Here's how the part is built. I have some questions about the finished solid (model axes, mm). A direction names the side the tool comes from. Round coordinates to 2 decimals unless told otherwise and drop trailing zeros. Order: outer loops, then holes, each group sorted by start corner. A loop starts at its lowest first (then second) coordinate and runs counter-clockwise, first axis right, second up. Notation, with made-up numbers: (74, -18) -> (78, -18) arc R26 ccw to (78, 6) -> close; hole circle Ø9 at (53, 59.5). An arc over 180 degrees is marked (long way). One line per item, written item: value.
```python
from build123d import *

# Parameters (mm, degrees)
SKETCH1_W           = 82.0674
SKETCH1_H           = 79.121
SKETCH1_R           = 12.7
SKETCH1_W_2         = 28.575
SKETCH1_H_2         = 58.801
BOSS_EXTRUDE1_DEPTH = 25.4


with BuildPart() as part:
    # Sketch1 → Boss-Extrude1 (new body)
    with BuildSketch(Plane(origin=(0, 0, 0), x_dir=(1, 0, 0), z_dir=(0, 1, 0))):
        with Locations((-41.0337, 39.5605)):
            Rectangle(SKETCH1_W, SKETCH1_H)
        with Locations(Location((-23.495, 54.61, 0), (0, 0, 270))):
            Circle(SKETCH1_R, mode=Mode.SUBTRACT)
        with Locations((-61.4299, 39.5605)):
            Rectangle(SKETCH1_W_2, SKETCH1_H_2, mode=Mode.SUBTRACT)
    extrude(amount=BOSS_EXTRUDE1_DEPTH)


solid = part.part
```
Q1. I want a section at A-A on x = -62. Write out the boundary of the cut face in (y, z).
Answers:
outline: (0, -79.12) -> (25.4, -79.12) -> (25.4, -68.96) -> (0, -68.96) -> close; (0, -10.16) -> (25.4, -10.16) -> (25.4, 0) -> (0, 0) -> close
Q2. Which directions (+Z, -Z, +X, -X, +Y, -Y) give clear straight access to the entire face, cutting with the end or side of a thin tool? Please do faces 5 (the face through (-42, 13, 0)), 6 (the face through (-62, 13, -10.16)).
Answers:
face 5: +Z, +X, -X, +Y, -Y
face 6: +Y, -Y
Q3. I want a section at D-D on y = 16. Write out the boundary of the cut face in (x, z) (3 decimals), then the cut area to 3 significant figures.
Answers:
outline: (-82.067, -79.121) -> (0, -79.121) -> (0, 0) -> (-82.067, 0) -> close; hole (-75.717, -68.961) -> (-47.142, -68.961) -> (-47.142, -10.16) -> (-75.717, -10.16) -> close; hole circle Ø25.4 at (-23.495, -54.61)
area: 4,310 mm2
Q4. For P1, Ø12, axis at x = -38.5, z = -39.5, coming from the -Y side; P2, Ø20.5, axis at x = -23.495, z = -54.61, coming from the +Y side, each with a flat end and sliding along its axis, tell me the tip position at first contact or that it passes through.
Answers:
P1: y = 0
P2: through
Q5. I want a section at C-C on z = -54.61. Write out the boundary of the cut face in (x, y) (3 decimals), then the cut area to 3 significant figures.
Answers:
outline: (-82.067, 0) -> (-75.717, 0) -> (-75.717, 25.4) -> (-82.067, 25.4) -> close; (-47.142, 0) -> (-36.195, 0) -> (-36.195, 25.4) -> (-47.142, 25.4) -> close; (-10.795, 0) -> (0, 0) -> (0, 25.4) -> (-10.795, 25.4) -> close
area: 714 mm2
Q6. I need wall thicknesses on line 1 along X through (y, z) = (8.5, -54.61) (3 decimals); line 2 along Z through (x, y) = (-50.5, 11); line 3 along X through (y, z) = (13.5, -28). Which ranges of each line are inside material? Lowest first, please.
Answers:
line 1: -82.067 to -75.717, -47.142 to -36.195, -10.795 to 0
line 2: -79.12 to -68.96, -10.16 to 0
line 3: -82.07 to -75.72, -47.14 to 0
Q7. If we mould it in two halves opening along X, with no side actions, what happens to faces 1 (the face through (-32, 0, -40)), 2 (the face through (-47.142, 13, -39)), 3 (the face through (-82.067, 13, -39)), 4 (the face through (-75.717, 13, -39))? For each: pulls with the +X half, pulls with the -X half, needs draft (parallel to the pull), parting line crosses it, or undercut.
Answers:
face 1: needs draft
face 2: undercut
face 3: pulls with the -X half
face 4: undercut
Q8. I want a section at B-B on z = -21. Write out the boundary of the cut face in (x, y).
Answers:
outline: (-82.07, 0) -> (-75.72, 0) -> (-75.72, 25.4) -> (-82.07, 25.4) -> close; (-47.14, 0) -> (0, 0) -> (0, 25.4) -> (-47.14, 25.4) -> close
